Autodesk Inventor part; units mm, degrees
ref_plane "YZ Plane" through (0, 0, 0) normal (1, 0, 0) x (0, 1, 0)
ref_plane "XZ Plane" through (0, 0, 0) normal (0, 1, 0) x (-1, 0, 0)
ref_plane "XY Plane" through (0, 0, 0) normal (0, 0, 1) x (1, 0, 0)
sketch "Sketch1" plane through (0, 0, 0) normal (0, 0, 1) x (1, 0, 0)
  line L0 (0, 0) -> (0, 20.955)
  line L1 (4.445, 25.4) -> (505.6861, 25.4)
  line L2 (0, 0) -> (6.35, 0)
  line L3 (6.35, 0) -> (6.35, 15.875)
  line L4 (9.525, 19.05) -> (503.0416, 19.05)
  arc A0 (9.525, 19.05) -> (6.35, 15.875) centre (9.525, 15.875) ccw
  arc A1 (4.445, 25.4) -> (0, 20.955) centre (4.445, 20.955) ccw
  line L5 (509.3272, 23.5045) -> (519.0883, 9.5642)
  line L6 (505.6424, 17.6961) -> (513.8867, 5.922)
  arc A2 (509.3272, 23.5045) -> (505.6861, 25.4) centre (505.6861, 20.955) ccw
  arc A3 (505.6424, 17.6961) -> (503.0416, 19.05) centre (503.0416, 15.875) ccw
  line L7 (513.8867, 5.922) -> (519.0883, 9.5642)
  point P0 (0, 25.4)
  point P1 (508, 25.4)
  point P2 (0, 22.225)
  point P3 (3.175, 25.4)
  dimension "d0" = 508
  dimension "d1" = 25.4
  dimension "d2" = 6.35
  dimension "d3" = 6.35
  dimension "d26" = 90
  dimension "d33" = 4.445
  dimension "d35" = 6.35
  dimension "d36" = 125
  dimension "d37" = 4.445
  dimension "d38" = 3.175
  dimension "d41" = 17.018
extrude "Extrusion4" add sketch "Sketch1" along normal blind 1352.55
sketch "Sketch4" plane through (4.445, 25.4, 0) normal (0, 1, 0) x (1, 0, 0)
  line L0 (0, -1352.55) -> (501.2411, -1352.55)
  line L1 (0, 0) -> (501.2411, 0)
  line L2 (-4.445, 0) -> (-4.445, -1352.55)
  line L3 (514.6433, 0) -> (514.6433, -1352.55)
  line L4 (46.355, 0) -> (109.855, 0)
  line L5 (109.855, 0) -> (109.855, -88.9)
  line L6 (109.855, -88.9) -> (46.355, -88.9)
  line L7 (46.355, -88.9) -> (46.355, 0)
  line L8 (46.355, -1352.55) -> (109.855, -1352.55)
  line L9 (109.855, -1352.55) -> (109.855, -1263.65)
  line L10 (109.855, -1263.65) -> (46.355, -1263.65)
  line L11 (46.355, -1263.65) -> (46.355, -1352.55)
  dimension "d44" = 63.5
  dimension "d45" = 88.9
  dimension "d46" = 50.8
  dimension "d47" = 88.9
  dimension "d48" = 50.8
  dimension "d49" = 63.5
extrude "Extrusion5" cut sketch "Sketch4" against normal blind 12.7
sketch "Sketch5" plane through (505.6861, 25.4, 1352.55) normal (0, 1, 0) x (1, 0, 0)
  line L0 (-391.3861, 0) -> (0, 0)
  line L1 (-391.3861, 1352.55) -> (0, 1352.55)
  line L2 (13.4023, 1352.55) -> (13.4023, 0)
  line L3 (-69.5716, 0) -> (14.7564, 0)
  line L4 (14.7564, 0) -> (14.7564, 60.325)
  line L5 (14.7564, 60.325) -> (-69.5716, 60.325)
  line L6 (-69.5716, 60.325) -> (-69.5716, 0)
  line L7 (14.7422, 1352.55) -> (-69.5858, 1352.55)
  line L8 (-69.5858, 1352.55) -> (-69.5858, 1292.225)
  line L9 (-69.5858, 1292.225) -> (14.7422, 1292.225)
  line L10 (14.7422, 1292.225) -> (14.7422, 1352.55)
  point P0 (-505.6861, 1352.55)
  dimension "d52" = 84.328
  dimension "d53" = 60.325
  dimension "d55" = 60.325
  dimension "d56" = 84.328
extrude "Extrusion6" cut sketch "Sketch5" against normal blind 50.8
properties part number "GE-12060"
The model under review builds one solid part; all positions refer to its coordinate system, in mm. A direction names the side the tool comes from. Round coordinates to 2 decimals unless told otherwise and drop trailing zeros. Loops run counter-clockwise (first coordinate to the right, second up) from the corner with the lowest first, then second, coordinate; pieces in that order, holes last. Notation, with made-up numbers: (20.25, -5) -> (72.25, -5) arc R13 ccw to (72.25, 7) -> close; hole circle Ø9 at (70, 89). An arc over 180 degrees is marked (long way). Answer as a JSON object with one key per item and string values. Group by question number.
1) For line 1 (X direction, y = 3.75, z = 1147); line 2 (Y direction, x = 129, z = 308); line 3 (X direction, y = 15, z = 1251), list the stretches that pass through material, from the lowest coordinate up. Write a range as [from, to].
2) For pin 1 Ø10 at (y, z) = (11, 937) entering from +X; pin 2 Ø5 at (x, y) = (69.5, 23) entering from +Z; pin 3 Ø3 at (y, z) = (21.5, 1310.5) entering from -X; pin 4 Ø3 at (y, z) = (23.5, 1311.5) entering from +X, all flat-tipped, find the tip position at first contact; note any pin that passes through.
3) We need section B-B on x = 463. Write out the cut boundary in (y, z) (3 decimals).
4) For faces 1 (the face through (252, 25.4, 667)), 2 (the face through (253, 19.05, 667)), list the 3-axis set-ups (+Z, -Z, +X, -X, +Y, -Y) from which the entire face can be reached by the end or side of a thin tool; tool diameter is ignored.
5) We need section C-C on x = 145. Write out the cut boundary in (y, z).
Result set:
{
 "1": {"line 1": "[0, 6.35]", "line 2": "[19.05, 25.4]", "line 3": "[0, 6.35], [507.53, 515.28]"},
 "2": {"pin 1": "x = 519.09", "pin 2": "z = 1263.65", "pin 3": "x = 0", "pin 4": "x = 436.11"},
 "3": {"outline": "(19.05, 60.325) -> (25.4, 60.325) -> (25.4, 1292.225) -> (19.05, 1292.225) -> close"},
 "4": {"face 1": "+Z, -Z, +X, -X, +Y", "face 2": "+Z, -Z, -Y"},
 "5": {"outline": "(19.05, 0) -> (25.4, 0) -> (25.4, 1352.55) -> (19.05, 1352.55) -> close"}
}
